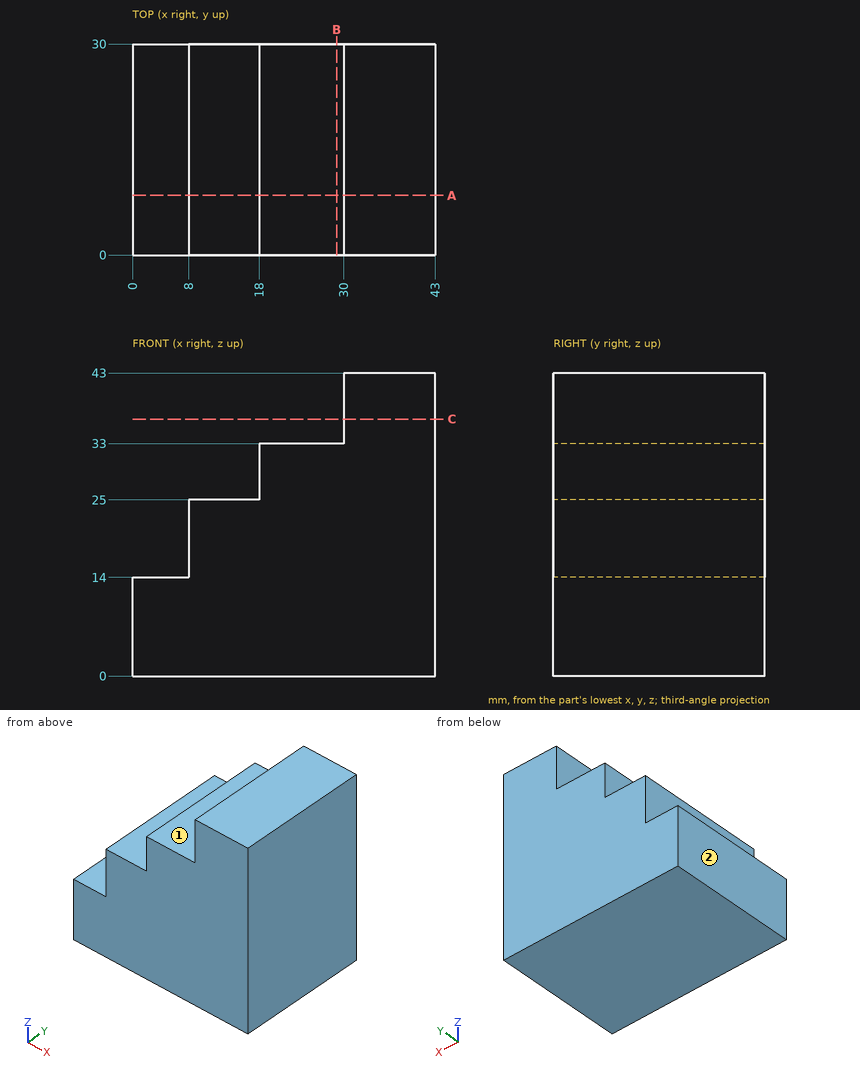
Job drawing, mm, ordinate dimensions from the low corner. One solid piece. A direction names the side the tool comes from. Coordinates: 2 decimals unless noted, no trailing zeros. Loops run counter-clockwise (first coordinate to the right, second up) from the corner with the lowest first, then second, coordinate; pieces in that order, holes last. Notation, with made-up numbers: (62, 76) - (77, 76) arc R13 cw to (77, 94) - close; hole circle Ø10 at (75.5, 14.5). An arc over 180 degrees is marked (long way). Write item = value, one per line. Start each with the question number.
Q1. Flat gauge pins, fed straight in: pin 1 Ø3 at (y, z) = (21.5, 22.5) entering from -X; pin 2 Ø12 at (x, y) = (5, 22.5) entering from -Z; pin 3 Ø8 at (x, y) = (14.5, 10) entering from +Z; pin 4 Ø3 at (y, z) = (11.5, 39) entering from -X. Where does each tip first touch, or does it go through?
Q2. Cut at B-B, the plane x = 29. List the corners of the cut face in (y, z), then the cut area to 3 significant figures.
Q3. Drill centre lines: L1, parallel to Z at x = 10.5, y = 13.25; L2, parallel to X at y = 5.25, z = 39; L3, parallel to Z at x = 18.5, y = 3.5. Where is each one in solid material? Low to high.
Q4. Cut at A-A, the plane y = 8.5. List the corners of the cut face in (x, z).
Q5. Cut at C-C, the plane z = 36.5. List the corners of the cut face in (x, y), then the cut area to 3 significant figures.
Q6. Which spindle directions (+Z, -Z, +X, -X, +Y, -Y) get a long thin tool onto all of the face, cutting with end or side? Do the marked faces 1 and 2. Say none if no direction does.
Computed:
q1.pin_1 = 8
q1.pin_2 = 0
q1.pin_3 = 33
q1.pin_4 = 30
q2.outline = (0, 0) - (30, 0) - (30, 33) - (0, 33) - close
q2.area = 990 mm²
q3.L1 = 0 to 25
q3.L2 = 30 to 43
q3.L3 = 0 to 33
q4.outline = (0, 0) - (43, 0) - (43, 43) - (30, 43) - (30, 33) - (18, 33) - (18, 25) - (8, 25) - (8, 14) - (0, 14) - close
q5.outline = (30, 0) - (43, 0) - (43, 30) - (30, 30) - close
q5.area = 390 mm²
q6.face_1 = +Z, -X, +Y, -Y
q6.face_2 = +Z, -Z, -X, +Y, -Y
